Source: CAD feature listing. Evaluate the final solid. Frame: model axes, mm. A direction names the side the tool comes from. Give positions to 0.01 mm unless a question says otherwise; leave off trailing zeros. Loops run counter-clockwise (first coordinate to the right, second up) from the corner with the lowest first, then second, coordinate; pieces in that order, holes last. Notation, with made-up numbers: (-19, 53) -> (0, 53) arc R24 cw to (0, 75) -> close; hole circle Ø8 at (19, -10.75). An arc over 180 degrees is marked (long way). Put each result on its own line as item: value.
```python
from build123d import *


# Not quite as in the source:
# - a feature names something its author has since deleted; it is built from what else it names


with BuildPart() as f1:
    # F0 (on Front) → F1 (revolve)
    with BuildSketch(Plane.XZ):
        with BuildLine():
            Line((-15, -25), (-12, -25))
            Line((-12, -25), (-12, -30))
            Line((-12, -30), (-9, -30))
            Line((-9, -30), (-9, -7.2415010072))
            ThreePointArc((-9, -7.2415010072), (-4.9914312836, -4.0779872119), (0, -3))
            Line((0, -3), (0, 0))
            Line((0, 0), (-15, 0))
            Line((-15, 0), (-15, -3))
            Line((-15, -3), (-15, -25))
        make_face()
    revolve(axis=Axis((0, 0, -1.5), (0, 0, -1)))


solid = f1.part
```
(1) First-contact query: P1, Ø3, axis at y = -7.5, z = -4.5, coming from the +X side; P2, Ø8, axis at y = 10.5, z = -8, coming from the +X side; P3, Ø2, axis at x = -2.5, z = -18.5, coming from the +Y side. Flat tips, straight axial feed; report the tip coordinate or a pass-through.
Calculated:
P1: stops at x = 13.75
P2: stops at x = 13.52
P3: stops at y = 14.92
(2) Line query: probe 1 along Y at (x, z) = (0, -18.5); probe 2 along X at (y, z) = (1, -26.5); probe 3 along Y at (x, z) = (-2.75, -5.5). Output: solid intervals per line, ascending. Write a range as from..to.
Calculated:
probe 1: y = -15..-9, 9..15
probe 2: x = -11.96..-8.94, 8.94..11.96
probe 3: y = -14.75..-6.72, 6.72..14.75
(3) Section A-A on z = -11.25. Return loops of the section in (x, y), then the cut area to 3 significant figures.
Calculated:
outline: circle Ø30 at (0, 0); hole circle Ø18 at (0, 0)
area: 452 mm²
(4) Draft query along X for faces 1 (the flat face through (7, 10, -25)), 2 (the cylindrical face through (14.985, 0.66, -12.675)), 3 (the cylindrical face through (1.172, 8.923, -18.461)). Return one class per face: released by +X, released by -X, zero draft, split by the parting line, or undercut.
Calculated:
face 1: zero draft
face 2: split by the parting line
face 3: undercut
(5) Section B-B on y = 10. Return loops of the section in (x, z).
Calculated:
outline: (-11.18, -25) -> (-6.63, -25) -> (-6.63, -30) -> (6.63, -30) -> (6.63, -25) -> (11.18, -25) -> (11.18, 0) -> (-11.18, 0) -> close
(6) Reachability of faces 4 (the flat face through (-2, 9, -30)), 5 (the cylindrical face through (11.99, 0.53, -27.54)) from +Z, -Z, +X, -X, +Y, -Y: full face, straight path, thin tool, end or side. Return the list, or none.
Calculated:
face 4: -Z, +X, -X, +Y, -Y
face 5: -Z
